Input: part model. Units: mm. Frame: model coordinates. Face numbers are marked on the shaded views. Give positions to 0.01 mm unless a question says otherwise; leave off trailing zeros. Loops run counter-clockwise (first coordinate to the right, second up) from the corner with the lowest first, then second, coordinate; pieces in that order, holes last.
from build123d import *

# Parameters (mm, degrees)
BOSS_EXTRUDE1_DEPTH = 19.05
SHELL1_T            = -1.5875
SKETCH2_W           = 15.875
SKETCH2_H           = 15.875
CUT_EXTRUDE1_DEPTH  = 221.078395706
SKETCH3_R           = 3.25
CUT_EXTRUDE2_DEPTH  = 2.54
SKETCH7_R           = 1.5875
CUT_EXTRUDE3_DEPTH  = 20.05
CUT_EXTRUDE4_DEPTH  = 19.05


with BuildPart() as part:
    # Sketch1 → Boss-Extrude1 (new body)
    with BuildSketch(Plane.XY):
        Polygon((-220.570309856, 200.660746496), (-205.600965293, 212.442988361), (-75.21082199, 46.782241865), (-90.180166553, 35), align=None)
    extrude(amount=BOSS_EXTRUDE1_DEPTH)

    # Shell1
    shell1_openings = [part.faces().sort_by_distance(p)[0] for p in [
        (-82.695494272, 40.891120932, 9.525),
    ]]
    offset(amount=SHELL1_T, openings=shell1_openings, kind=Kind.INTERSECTION)

    # Sketch2 → Cut-Extrude1 (cut, through all)
    with BuildSketch(Plane(origin=(-181.896970564, 231.100197958, 0), x_dir=(0.785792366, 0.618490387, 0), z_dir=(-0.618490387, 0.785792366, 0))):
        with Locations((-39.690722867, -9.525)):
            Rectangle(SKETCH2_W, SKETCH2_H)
    extrude(amount=-CUT_EXTRUDE1_DEPTH, mode=Mode.SUBTRACT)

    # Sketch3 → Cut-Extrude2 (cut)
    with BuildSketch(Plane.XY.offset(19.05)):
        with Locations((-203.807891879, 194.764486582)):
            Circle(SKETCH3_R)
    extrude(amount=-CUT_EXTRUDE2_DEPTH, mode=Mode.SUBTRACT)

    # Sketch7 → Cut-Extrude3 (cut, through all)
    with BuildSketch(Plane.XY.offset(19.05)):
        with Locations((-106.259978001, 70.829810058)):
            Circle(SKETCH7_R)
        with Locations((-90.550322182, 50.870683974)):
            Circle(SKETCH7_R)
    extrude(amount=-CUT_EXTRUDE3_DEPTH, mode=Mode.SUBTRACT)

    # Sketch9 → Cut-Extrude4 (cut)
    with BuildSketch(Plane.XY.offset(19.05)):
        with BuildLine():
            Line((-197.681280238, 189.405883238), (-195.825809078, 187.048506142))
            ThreePointArc((-195.825809078, 187.048506142), (-196.076762046, 184.942082013), (-198.183186175, 185.193034982))
            Line((-198.183186175, 185.193034982), (-200.038657334, 187.550412078))
            ThreePointArc((-200.038657334, 187.550412078), (-199.787704366, 189.656836206), (-197.681280238, 189.405883238))
        make_face()
        with BuildLine():
            Line((-209.432597583, 204.335938183), (-207.577126423, 201.978561086))
            ThreePointArc((-207.577126423, 201.978561086), (-207.828079392, 199.872136958), (-209.93450352, 200.123089926))
            Line((-209.93450352, 200.123089926), (-211.78997468, 202.480467023))
            ThreePointArc((-211.78997468, 202.480467023), (-211.539021711, 204.586891151), (-209.432597583, 204.335938183))
        make_face()
    extrude(amount=-CUT_EXTRUDE4_DEPTH, mode=Mode.SUBTRACT)


solid = part.part
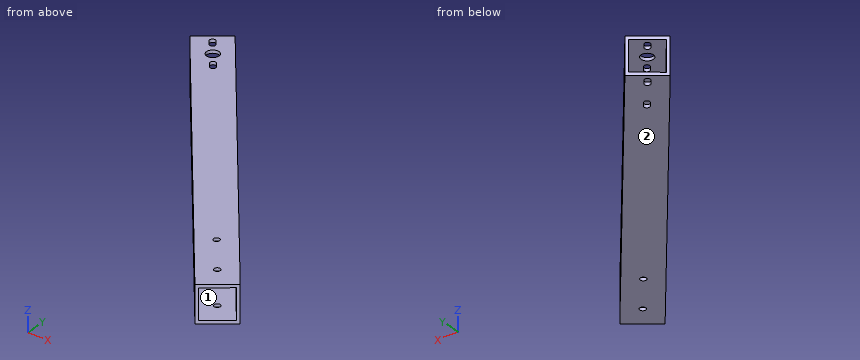
(1) Cut plane A-A (z = 4.25). Return the cut outline in (x, y).
Values follow:
outline: (-220.57, 200.66) - (-90.18, 35) - (-88.93, 35.98) - (-219.32, 201.64) - close; (-206.85, 211.46) - (-76.46, 45.8) - (-75.21, 46.78) - (-205.6, 212.44) - close
(2) Pin query (flat end, axial travel): pin 1 Ø4 at (y, z) = (125.5, 12) entering from +X; pin 2 Ø3 at (x, y) = (-90.55, 50.87) entering from +Z; pin 3 Ø1 at (y, z) = (102, 5) entering from +X; pin 4 Ø6 at (x, z) = (-139, 16) entering from +Y. Return the tip coordinate at first contact, or that it passes through.
Values follow:
pin 1: stops at x = -135.59
pin 2: passes through
pin 3: stops at x = -118.28
pin 4: stops at y = 131.64
(3) Ray query, probe 1 along Z at (x, y) = (-188.5, 172); probe 2 along X at (y, z) = (132, 5.75); probe 3 along X at (y, z) = (117, 16.25). Return the intervals inside material, ascending.
Values follow:
probe 1: z = 0 to 1.59, 17.46 to 19.05
probe 2: x = -166.53 to -164.51, -144.31 to -142.28
probe 3: x = -154.72 to -152.7, -132.5 to -130.48
(4) Cut plane C-C (y = 164.5). Return the cut outline in (x, z), and give its area (3 significant figures).
Values follow:
outline: (-192.11, 0) - (-167.87, 0) - (-167.87, 19.05) - (-192.11, 19.05) - close; hole (-190.09, 1.59) - (-169.89, 1.59) - (-169.89, 17.46) - (-190.09, 17.46) - close
area: 141 mm2
(5) Cut plane B-B (x = -160). Return the cut outline in (y, z), and give its area (3 significant figures).
Values follow:
outline: (123.71, 0) - (154.51, 0) - (154.51, 19.05) - (123.71, 19.05) - close; hole (126.27, 1.59) - (151.94, 1.59) - (151.94, 17.46) - (126.27, 17.46) - close
area: 179 mm2
(6) Mould query, pull axis X, two halves, no side actions, for the marked faces 1 and 2. Classes: +X half, -X half, draft (parallel to the pull), parting line (faces both ways), or undercut.
Values follow:
face 1: undercut
face 2: draft
